from build123d import *

# Parameters (mm, degrees)
F0_W     = 14
F0_H     = 28
F1_DEPTH = 8
F0_W_2   = 4
F2_DEPTH = 12
F3_D     = 5
F4_R     = 1.5


with BuildPart() as f1:
    # F0 (on Top) → F1 (new body)
    with BuildSketch(Plane.XY):
        with Locations((-7, 14)):
            Rectangle(F0_W, F0_H)
        with Locations((7, 14)):
            Rectangle(F0_W, F0_H)
    extrude(amount=F1_DEPTH)

    # F0 (on Top) → F2 (join)
    with BuildSketch(Plane.XY):
        with Locations((-16, 14)):
            Rectangle(F0_W_2, F0_H)
        with Locations((16, 14)):
            Rectangle(F0_W_2, F0_H)
    extrude(amount=F2_DEPTH)

    # F3 (through all)
    with Locations(Plane(origin=(0, 0, 0), x_dir=(1, 0, 0), z_dir=(0, 0, -1))):
        with Locations((0, -14)):
            Hole(F3_D / 2)

    # F4
    f4_edges = [f1.edges().sort_by_distance(p)[0] for p in [
        (-16, 0, 12),
        (-14, 14, 12),
        (-16, 28, 12),
        (-18, 14, 12),
        (14, 14, 12),
        (16, 0, 12),
        (18, 14, 12),
        (16, 28, 12),
        (0, 28, 8),
        (0, 0, 8),
    ]]
    fillet(f4_edges, radius=F4_R)


solid = f1.part
Here's how the part is built. I have some questions about the finished solid (model axes, mm). A direction names the side the tool comes from. Coordinates: 2 decimals unless noted, no trailing zeros. Loops run counter-clockwise (first coordinate to the right, second up) from the corner with the lowest first, then second, coordinate; pieces in that order, holes last.
1. If we mould it in two halves opening along X, with no side actions, what happens to faces 1 (the flat face through (16, 14, 12)), 2 (the flat face through (18, 14, 5)), 3 (the cylindrical face through (-14.45, 14.2, 11.57))? For each: pulls with the +X half, pulls with the -X half, needs draft (parallel to the pull), parting line crosses it, or undercut.
2. Imagine slicing it at A-A, the plane x = -2. Please give me the cut outline in (y, z).
3. I need wall thicknesses on L1, parallel to X at y = 21, z = 10.25; L2, parallel to X at y = 14, z = 6.25; L3, parallel to Y at x = 0, z = 3.5. Which ranges of each line are inside material? Lowest first, please.
4. Imagine slicing it at D-D, the plane z = 7. Please give me the cut outline in (x, y).
5. Imagine slicing it at B-B, the plane z = 10. Please give me the cut outline in (x, y).
6. For P1, Ø8, axis at x = -2.5, y = 5.5, coming from the +Z side, with a flat end and sliding along its axis, tell me the tip position at first contact or that it passes through.
7. For faces 4 (the cylindrical face through (14.43, 14.2, 11.55)), 5 (the flat face through (-16, 14, 12)), 6 (the cylindrical face through (0.2, 0.43, 7.55)), which set-ups out of +Z, -Z, +X, -X, +Y, -Y let a thin tool reach every point of the face, with its end or its side?
8. Imagine slicing it at C-C, the plane y = 14. Please give me the cut outline in (x, z).
Taken from the geometry:
1. face 1: needs draft
1. face 2: pulls with the +X half
1. face 3: undercut
2. outline: (0, 0) - (12.5, 0) - (12.5, 8) - (1.5, 8) arc R1.5 ccw to (0, 6.5) - close; (15.5, 0) - (28, 0) - (28, 6.5) arc R1.5 ccw to (26.5, 8) - (15.5, 8) - close
3. L1: x = -18 to -14, 14 to 18
3. L2: x = -18 to -2.5, 2.5 to 18
3. L3: y = 0 to 11.5, 16.5 to 28
4. outline: (-18, 0) - (-14, 0) - (-14, 0.09) - (14, 0.09) - (14, 0) - (18, 0) - (18, 28) - (14, 28) - (14, 27.91) - (-14, 27.91) - (-14, 28) - (-18, 28) - close; hole circle Ø5 at (0, 14)
5. outline: (-18, 0) - (-14, 0) - (-14, 28) - (-18, 28) - close; (14, 0) - (18, 0) - (18, 28) - (14, 28) - close
6. P1: stops at z = 8
7. face 4: +Z, +Y, -Y
7. face 5: +Z, +X, -X, +Y, -Y
7. face 6: +Z, -Y
8. outline: (-18, 0) - (-2.5, 0) - (-2.5, 8) - (-14, 8) - (-14, 10.5) arc R1.5 ccw to (-15.5, 12) - (-16.5, 12) arc R1.5 ccw to (-18, 10.5) - close; (2.5, 0) - (18, 0) - (18, 10.5) arc R1.5 ccw to (16.5, 12) - (15.5, 12) arc R1.5 ccw to (14, 10.5) - (14, 8) - (2.5, 8) - close
